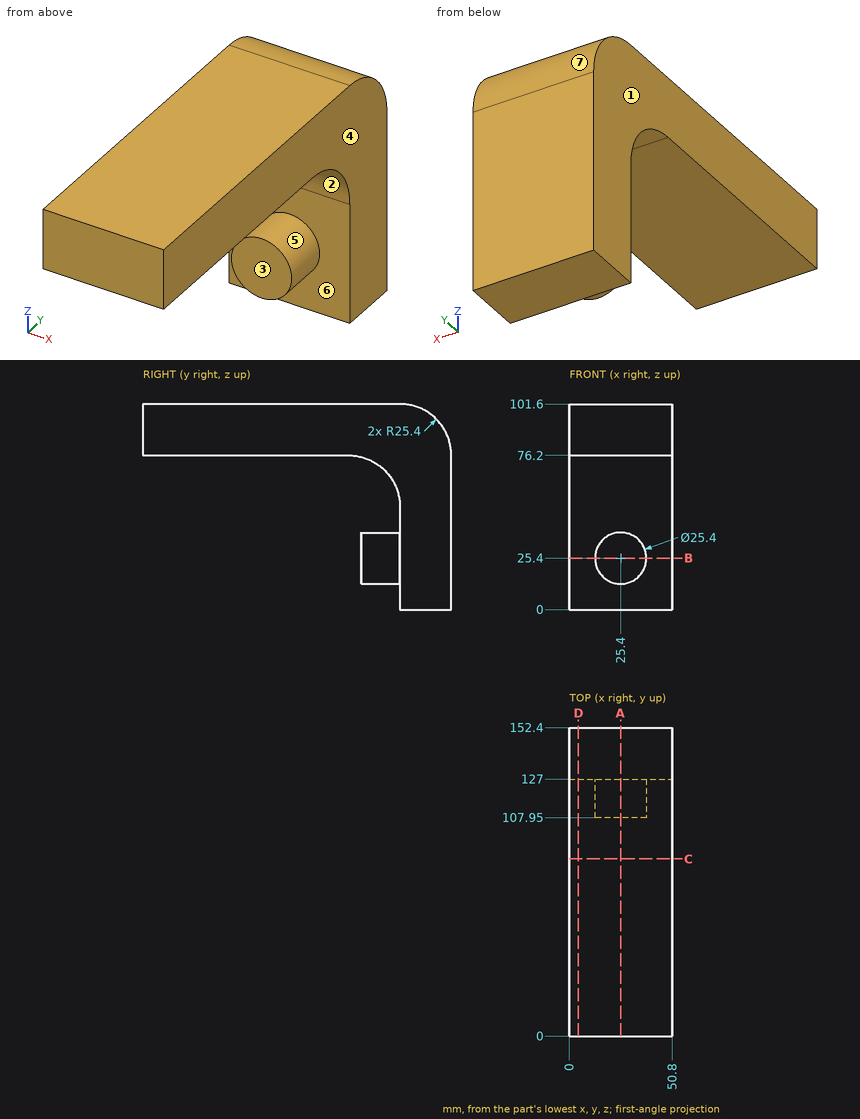
Answer from the drawing. Dimensions are ordinates in mm from the lowest x, y and z of the part. A direction names the side the tool comes from. Round coordinates to 2 decimals unless told otherwise and drop trailing zeros. Write each loop counter-clockwise with the first axis right and the second up, starting at its lowest first coordinate (ties: lowest second). Pieces come first, ordered by that corner, then holes. Notation, with made-up numbers: M 82.5,1.25 L 87.5,1.25 A4 cw 87.5,7.25 Z; hole C 51,87 d10. An arc over 180 degrees is marked long. One line per item, written item: value.
Q1. Straight lines are drawn through the part: line 1 (Z direction, x = 34.5, y = 52); line 2 (Y direction, x = 44.5, z = 10); line 3 (Z direction, x = 36.5, y = 121.5). For each, find the intervals that lie inside material, in ascending order. Write a range as [from, to].
Data:
line 1: [76.2, 101.6]
line 2: [127, 152.4]
line 3: [19.23, 31.57], [66.58, 101.6]
Q2. Find section D-D on x = 4.5. Write down the section's boundary in (y, z), plus the area to 3 significant figures.
Data:
outline: M 0,76.2 L 101.6,76.2 A25.4 cw 127,50.8 L 127,0 L 152.4,0 L 152.4,76.2 A25.4 ccw 127,101.6 L 0,101.6 Z
area: 5,810 mm2
Q3. Find section C-C on y = 87.5. Write down the section's boundary in (x, z), plus the area to 3 significant figures.
Data:
outline: M 0,76.2 L 50.8,76.2 L 50.8,101.6 L 0,101.6 Z
area: 1,290 mm2
Q4. For a pull along Z with two mould halves and no side action, classify the marked faces 4, 5, 6 and 7 as +Z half, -Z half, draft (parallel to the pull), parting line (faces both ways), or undercut.
Data:
face 4: draft
face 5: undercut
face 6: undercut
face 7: +Z half
Q5. Flat-ended cylindrical pins translate along their axes: pin 1 Ø20.5 at (x, z) = (24, 26) entering from -Y; pin 2 Ø3 at (y, z) = (108, 28) entering from +X. Find the tip coordinate at first contact, or state that the pin passes through.
Data:
pin 1: y = 107.95
pin 2: x = 38.05
Q6. Find section A-A on x = 25.4. Write down the section's boundary in (y, z).
Data:
outline: M 0,76.2 L 101.6,76.2 A25.4 cw 127,50.8 L 127,38.1 L 107.95,38.1 L 107.95,12.7 L 127,12.7 L 127,0 L 152.4,0 L 152.4,76.2 A25.4 ccw 127,101.6 L 0,101.6 Z
Q7. Find section B-B on z = 25.4. Write down the section's boundary in (x, y).
Data:
outline: M 0,127 L 12.7,127 L 12.7,107.95 L 38.1,107.95 L 38.1,127 L 50.8,127 L 50.8,152.4 L 0,152.4 Z
Q8. Which of the six approach directions +Z, -Z, +X, -X, +Y, -Y give full straight-line access (tool end or side, diameter ignored) to the marked faces 1, 2 and 3?
Data:
face 1: +Z, -Z, -X, +Y, -Y
face 2: +X, -X, -Y
face 3: -Z, +X, -X, -Y
